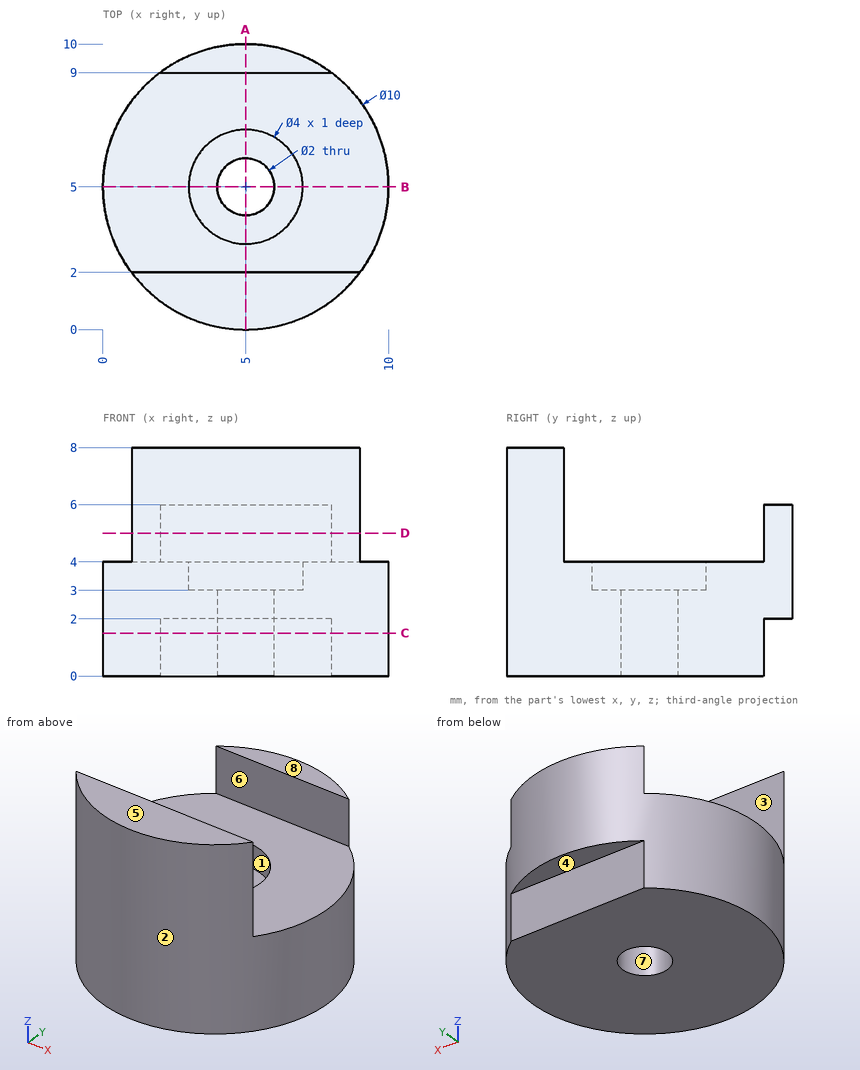
Geometry: see drawing. Coordinates: mm, zero at the bounding-box minimum. A direction names the side the tool comes from. Round coordinates to 2 decimals unless told otherwise and drop trailing zeros. Loops run counter-clockwise (first coordinate to the right, second up) from the corner with the lowest first, then second, coordinate; pieces in that order, holes last.
(1) Section query B-B (y = 5). Output: boundary loops of the cut face in (x, z).
From the geometry:
outline: (0, 0) - (4, 0) - (4, 3) - (3, 3) - (3, 4) - (0, 4) - close; (6, 0) - (10, 0) - (10, 4) - (7, 4) - (7, 3) - (6, 3) - close
(2) Contact query for flat-ended pins moving along their axis: pin 1 Ø0.5 at (x, y) = (4.5, 9.5) entering from +Z; pin 2 Ø1.2 at (x, z) = (5.5, 6.5) entering from +Y; pin 3 Ø2.5 at (x, y) = (5, 5) entering from +Z. Output: stop coordinate, or through.
From the geometry:
pin 1: stops at z = 6
pin 2: stops at y = 10
pin 3: stops at z = 3
(3) Material intervals for probe 1 along Y at (x, z) = (5, 3.65); probe 2 along X at (y, z) = (5, 0.7); probe 3 along Z at (x, y) = (6.5, 7), sorted ascending.
From the geometry:
probe 1: y = 0 to 3, 7 to 10
probe 2: x = 0 to 4, 6 to 10
probe 3: z = 0 to 4
(4) Section query D-D (z = 5). Output: boundary loops of the cut face in (x, y).
From the geometry:
outline: (1, 2) arc R5 ccw to (9, 2) - close; (2, 9) - (8, 9) arc R5 ccw to start
(5) Access query for the marked faces 4, 5, 6, 7 and 8. Directions: +Z, -Z, +X, -X, +Y, -Y. A direction counts if a zero-diameter tool reaches every point of the face in a straight line with its end or side. Return the directions, or none.
From the geometry:
face 4: -Z, +X, -X, +Y
face 5: +Z, +X, -X, +Y, -Y
face 6: +Z, +X, -X
face 7: +Z, -Z
face 8: +Z, +X, -X, +Y
(6) Section query C-C (z = 1.5). Output: boundary loops of the cut face in (x, y).
From the geometry:
outline: (2, 9) arc R5 ccw (long way) to (8, 9) - close; hole circle Ø2 at (5, 5)
(7) Section query A-A (x = 5). Output: boundary loops of the cut face in (y, z), and give its area (3 significant figures).
From the geometry:
outline: (0, 0) - (4, 0) - (4, 3) - (3, 3) - (3, 4) - (2, 4) - (2, 8) - (0, 8) - close; (6, 0) - (9, 0) - (9, 2) - (10, 2) - (10, 6) - (9, 6) - (9, 4) - (7, 4) - (7, 3) - (6, 3) - close
area: 38.0 mm2
(8) Pull-direction query (X, two-part tool) for the marked faces 1, 2 and 3; classes: +X half, -X half, draft (parallel to the pull), parting line (faces both ways), or undercut.
From the geometry:
face 1: undercut
face 2: parting line
face 3: draft
